Drawing for the job (mm, zero at the part's lowest x, y, z). A direction names the side the tool comes from. Coordinates: 2 decimals unless noted, no trailing zeros. Order: outer loops, then holes, each group sorted by start corner. A loop starts at its lowest first (then second) coordinate and runs counter-clockwise, first axis right, second up. Notation, with made-up numbers: (88, 30.5) - (139, 30.5) arc R32 cw to (139, 58.5) - close; hole circle Ø10 at (66.5, 54). An arc over 180 degrees is marked (long way). Answer as CSV lines item,"result". Start each with the question number.
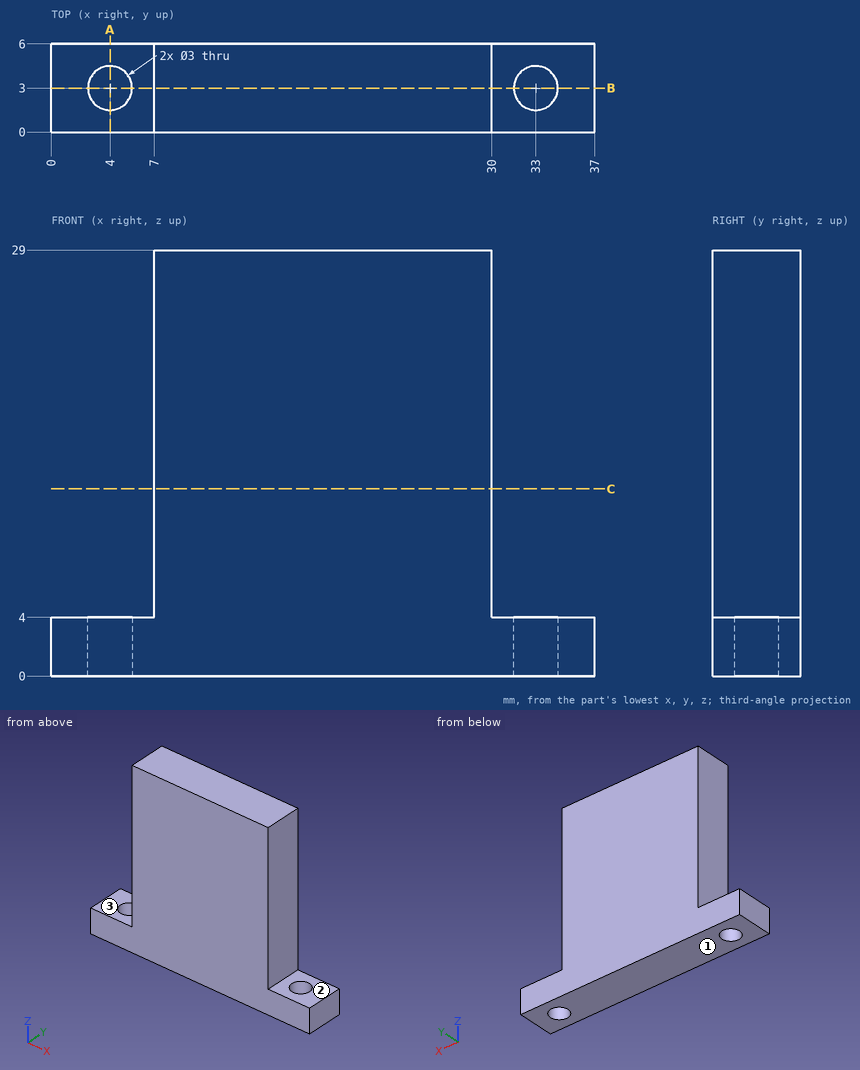
(1) Which spindle directions (+Z, -Z, +X, -X, +Y, -Y) get a long thin tool onto all of the face, cutting with end or side? Do the marked faces 1, 2 and 3. Say none if no direction does.
(2) Drop flat-ended pins along their axis: pin 1 Ø1.8 at (x, y) = (33, 3) entering from +Z; pin 2 Ø3 at (x, z) = (27, 14) entering from -Y; pin 3 Ø1.8 at (x, y) = (33.5, 2) entering from +Z; pin 4 Ø3 at (y, z) = (2.5, 15) entering from +X. Give the stop position or say it passes through.
(3) Band-saw the part on A-A on x = 4. List the corners of the cut face in (y, z).
(4) Band-saw the part on C-C on z = 12.75. List the corners of the cut face in (x, y).
(5) Probe L1, parallel to Y at x = 4, z = 3.15; L2, parallel to X at y = 3.35, z = 24.5; L3, parallel to Z at x = 34, y = 1.8. List the from-to ranges inside material, lowest first. Write a range as [from, to].
(6) Band-saw the part on B-B on y = 3. List the corners of the cut face in (x, z), plus the area to 3 significant figures.
Filled in:
1,face 1,"-Z, +X, -X, +Y, -Y"
1,face 2,"+Z, +X, +Y, -Y"
1,face 3,"+Z, -X, +Y, -Y"
2,pin 1,"passes through"
2,pin 2,"stops at y = 0"
2,pin 3,"stops at z = 4"
2,pin 4,"stops at x = 30"
3,outline,"(0, 0) - (1.5, 0) - (1.5, 4) - (0, 4) - close; (4.5, 0) - (6, 0) - (6, 4) - (4.5, 4) - close"
4,outline,"(7, 0) - (30, 0) - (30, 6) - (7, 6) - close"
5,L1,"y = [0, 1.5], [4.5, 6]"
5,L2,"x = [7, 30]"
5,L3,"z = [0, 4]"
6,outline,"(0, 0) - (2.5, 0) - (2.5, 4) - (0, 4) - close; (5.5, 0) - (31.5, 0) - (31.5, 4) - (30, 4) - (30, 29) - (7, 29) - (7, 4) - (5.5, 4) - close; (34.5, 0) - (37, 0) - (37, 4) - (34.5, 4) - close"
6,area,"699 mm^2"
